Could you check a few things on this model? Use its own coordinates, in mm. Face numbers are marked on the shaded views. A direction names the side the tool comes from. Coordinates: 2 decimals unless noted, no trailing zeros. Write each loop counter-clockwise with the first axis right and the second up, starting at its lowest first coordinate (ties: lowest second). Pieces come first, ordered by that corner, then holes. Notation, with made-up numbers: M 19,52 L 74,52 A24 cw 74,72 Z; hole C 64.5,40 d8. An arc over 180 degrees is marked long. Write item = value, one per line.
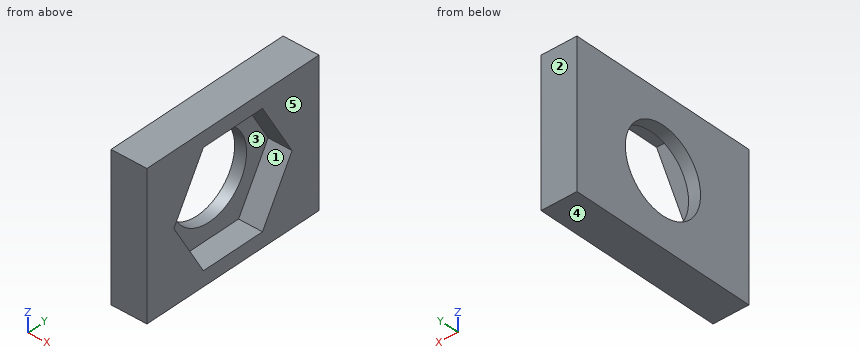
```python
from build123d import *

# Parameters (mm, degrees)
SKETCH1_W           = 12
SKETCH1_H           = 12
BOSS_EXTRUDE1_DEPTH = 3
SKETCH2_R           = 3.5
CUT_EXTRUDE1_DEPTH  = 3
CUT_EXTRUDE2_DEPTH  = 2
SKETCH4_W           = 3
SKETCH4_H           = 12
BOSS_EXTRUDE2_DEPTH = 2
SKETCH5_W           = 3
SKETCH5_H           = 12
BOSS_EXTRUDE3_DEPTH = 2


with BuildPart() as part:
    # Sketch1 → Boss-Extrude1 (new body)
    with BuildSketch(Plane(origin=(0, 0, 0), x_dir=(0, 0, -1), z_dir=(1, 0, 0))):
        with Locations((6, 6)):
            Rectangle(SKETCH1_W, SKETCH1_H)
    extrude(amount=BOSS_EXTRUDE1_DEPTH)

    # Sketch2 → Cut-Extrude1 (cut)
    with BuildSketch(Plane(origin=(3, 0, 0), x_dir=(0, 0, -1), z_dir=(1, 0, 0))):
        with Locations((6, 6)):
            Circle(SKETCH2_R)
    extrude(amount=-CUT_EXTRUDE1_DEPTH, mode=Mode.SUBTRACT)

    # Sketch3 → Cut-Extrude2 (cut)
    with BuildSketch(Plane(origin=(3, 0, 0), x_dir=(0, 0, -1), z_dir=(1, 0, 0))):
        Polygon((6, 11.5), (1.236860279, 8.75), (1.236860279, 3.25), (6, 0.5), (10.763139721, 3.25), (10.763139721, 8.75), align=None)
    extrude(amount=-CUT_EXTRUDE2_DEPTH, mode=Mode.SUBTRACT)

    # Sketch4 → Boss-Extrude2 (add)
    with BuildSketch(Plane(origin=(0, 12, 0), x_dir=(1, 0, 0), z_dir=(0, 1, 0))):
        with Locations((1.5, 6)):
            Rectangle(SKETCH4_W, SKETCH4_H)
    extrude(amount=BOSS_EXTRUDE2_DEPTH)

    # Sketch5 → Boss-Extrude3 (add)
    with BuildSketch(Plane.XZ):
        with Locations((1.5, -6)):
            Rectangle(SKETCH5_W, SKETCH5_H)
    extrude(amount=BOSS_EXTRUDE3_DEPTH)


solid = part.part
```
Item 1: If we mould it in two halves opening along Z, with no side actions, what happens to the marked faces 3, 4 and 5? For each: pulls with the +Z half, pulls with the -Z half, needs draft (parallel to the pull), parting line crosses it, or undercut.
Numbers:
face_3 = undercut
face_4 = pulls with the -Z half
face_5 = needs draft
Item 2: Imagine slicing it at B-B (y = 6). Write out the boundary of the cut face in (x, z), and give its area (3 significant figures).
Numbers:
outline = M 0,-12 L 3,-12 L 3,-10.76 L 1,-10.76 L 1,-9.5 L 0,-9.5 Z; M 0,-2.5 L 1,-2.5 L 1,-1.24 L 3,-1.24 L 3,0 L 0,0 Z
area = 9.95 mm²
Item 3: Imagine slicing it at C-C (z = -9). Write out the boundary of the cut face in (x, y), and give its area (3 significant figures).
Numbers:
outline = M 0,-2 L 3,-2 L 3,2.23 L 1,2.23 L 1,4.2 L 0,4.2 Z; M 0,7.8 L 1,7.8 L 1,9.77 L 3,9.77 L 3,14 L 0,14 Z
area = 29.3 mm²
Item 4: For the marked faces 1 and 2, which set-ups out of +Z, -Z, +X, -X, +Y, -Y let a thin tool reach every point of the face, with its end or its side?
Numbers:
face_1 = +X
face_2 = +Z, -Z, +X, -X, +Y
Item 5: Imagine slicing it at D-D (x = 0.75). Write out the boundary of the cut face in (y, z).
Numbers:
outline = M -2,-12 L 14,-12 L 14,0 L -2,0 Z; hole C 6,-6 d7
Item 6: Imagine slicing it at A-A (x = 1.5). Write out the boundary of the cut face in (y, z).
Numbers:
outline = M -2,-12 L 14,-12 L 14,0 L -2,0 Z; hole M 0.5,-6 L 3.25,-10.76 L 8.75,-10.76 L 11.5,-6 L 8.75,-1.24 L 3.25,-1.24 Z
Item 7: If I drill on line 1 along Z through (x, y) = (2.6, 5.25); line 2 along Y through (x, z) = (0.6, -6); line 3 along X through (y, z) = (7, -9.75), over which ranges is the centre line in solid material (lowest first)?
Numbers:
line_1 = -12 to -10.76, -1.24 to 0
line_2 = -2 to 2.5, 9.5 to 14
line_3 = 0 to 1
Item 8: I'm going to push a flat-ended pin straight in: P1, Ø5.5, axis at y = 6, z = -6, coming from the +X side. Where does the tip first touch, or does it pass through?
Numbers:
P1 = through
